Geometry: final body of the model. Coordinates: model frame, mm. Give positions to 0.01 mm unless a question says otherwise; leave off trailing zeros. Loops run counter-clockwise (first coordinate to the right, second up) from the corner with the lowest first, then second, coordinate; pieces in that order, holes last.
1. Section A-A, the plane x = 0.45. Output: boundary loops of the cut face in (y, z).
2. Section B-B, the plane z = -23.5. Output: boundary loops of the cut face in (x, y), then the cut area to 3 significant figures.
3. Material intervals for line 1 along Y through (x, z) = (0.55, 61); line 2 along Z through (x, y) = (-0.4, 67), sorted ascending.
4. First-contact query: P1, Ø0.6, axis at x = -0.5, z = -35, coming from the -Y side; P2, Ø0.6, axis at x = 0.5, z = -71.5, coming from the -Y side; P3, Ø0.6, axis at x = 0, y = -1.5, coming from the +Z side. Flat tips, straight axial feed; report the tip coordinate or a pass-through.
Autodesk Inventor part; units mm, degrees
ref_plane "Work Plane2" through (0, 0, 0) normal (0, -1, 0) x (1, 0, 0)
ref_plane "Work Plane4" through (1, 0, -70) normal (0, 0, 1) x (1, 0, 0)
ref_plane "YZ Plane" through (0, 0, 0) normal (1, 0, 0) x (0, 1, 0)
sketch "Sketch1" plane through (0, 0, 0) normal (0, 1, 0) x (-1, 0, 0)
  line L0 (1, 75) -> (-1, 75)
  line L1 (-1, 75) -> (-1, -70.101)
  line L2 (-1, -75) -> (0, -75) construction
  line L3 (1, -75) -> (1, -70.101) construction
  line L4 (0, 75) -> (0, -75) construction
  arc A0 (1, -70.101) -> (-1, -70.101) centre (0, -75) ccw
  arc A1 (-1, -70.101) -> (1, -70.101) centre (0, -75) ccw construction
  line L5 (1, -70.101) -> (1, 75)
  line L6 (0, -75) -> (1, -75) construction
  line L7 (-1, -70.101) -> (-1, -75) construction
  point P0 (0, 0)
  point P1 (0, 0)
  dimension "d0" = 2
  dimension "d1" = 150
  dimension "d18" = 10
extrude "Extrusion1" add sketch "Sketch1" along normal blind 130
ref_plane "Work Plane2" through (0, 0, 0) normal (0, -1, 0) x (1, 0, 0)
sketch "Sketch2" plane through (0, 0, 0) normal (0, -1, 0) x (1, 0, 0)
  line L0 (1, 15) -> (-1, 15)
  line L1 (-1, 15) -> (-1, -15)
  line L2 (-1, -15) -> (1, -15)
  line L3 (1, -15) -> (1, 15)
  line L4 (0, 15) -> (0, -15) construction
  point P0 (0, 0)
  point P1 (0, 0)
  dimension "d5" = 2
  dimension "d6" = 30
extrude "Extrusion2" add sketch "Sketch2" along normal blind 2
ref_plane "Work Plane4" through (1, 0, -70) normal (0, 0, 1) x (1, 0, 0)
sketch "Sketch4" plane through (1, 0, -70) normal (0, 0, 1) x (1, 0, 0)
  line L0 (0, 115) -> (-2, 115)
  line L1 (-2, 115) -> (-2, 95)
  line L2 (-2, 95) -> (0, 95)
  line L3 (0, 95) -> (0, 115)
  line L4 (-1, 115) -> (-1, 95) construction
  line L5 (-1, 0) -> (-1, 130) construction
  line L6 (-2, 130) -> (0, 130) construction
  line L7 (-2, 35) -> (0, 35)
  line L8 (0, 35) -> (0, 15)
  line L9 (0, 15) -> (-2, 15)
  line L10 (-2, 15) -> (-2, 35)
  line L11 (-1, 35) -> (-1, 15) construction
  line L12 (-2, 0) -> (0, 0) construction
  dimension "d20" = 2
  dimension "d21" = 20
  dimension "d22" = 15
  dimension "d23" = 2
  dimension "d24" = 20
  dimension "d25" = 15
extrude "Extrusion4" add sketch "Sketch4" against normal blind 2
properties part number "sidePlate" material "Aluminum 6061"
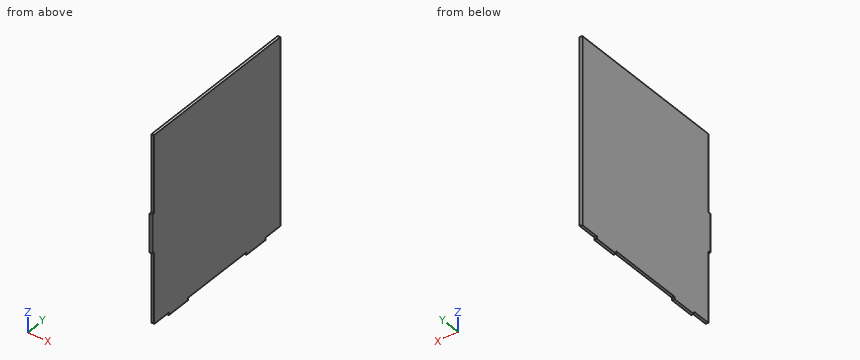
Answers below:
1. outline: (-2, -15) - (0, -15) - (0, -70.02) - (15, -70.02) - (15, -72) - (35, -72) - (35, -70.02) - (95, -70.02) - (95, -72) - (115, -72) - (115, -70.02) - (130, -70.02) - (130, 75) - (0, 75) - (0, 15) - (-2, 15) - close
2. outline: (-1, 0) - (1, 0) - (1, 130) - (-1, 130) - close
2. area: 260 mm2
3. line 1: y = 0 to 130
3. line 2: z = -70.02 to 75
4. P1: stops at y = 0
4. P2: stops at y = 15
4. P3: stops at z = 15
